Can you work these out from the model? Positions are in its coordinate system, mm. Give positions to 0.01 mm unless a question says otherwise; leave off trailing zeros. Order: outer loops, then holes, each group sorted by start corner. A loop starts at its lowest first (then second) coordinate and runs counter-clockwise, first axis right, second up. Notation, with made-up numbers: (5.5, 26.25) - (61.5, 26.25) arc R21 cw to (61.5, 35.25) - close; hole circle Ø4 at (-39.75, 7). An arc over 180 degrees is marked (long way). Answer as a JSON object with one key per item and string values.
```python
from build123d import *

# Parameters (mm, degrees)
F1_DEPTH = 31.75
F3_D     = 12.7


with BuildPart() as f1:
    # F0 (on Top) → F1 (new body)
    with BuildSketch(Plane.XY):
        with BuildLine():
            Line((45.9964759648, 36.0500998795), (-9.8253758624, 36.0500998795))
            add(Edge.make_bspline(
                [(-42.9035240352, 4.3000998795), (-34.7231067307, 4.914947889), (-18.4671684559, 14.0682512449), (-11.2220877593, 28.5159185869), (-9.8253758624, 36.0500998795)],
                knots=[0, 0, 0, 0, 0.5112036525, 1, 1, 1, 1], degree=3))
            Line((-42.9035240352, 4.3000998795), (-42.9035240352, -27.4499001205))
            Line((-42.9035240352, -27.4499001205), (-22.798109327, -27.4499001205))
            Line((-22.798109327, -27.4499001205), (45.9964759648, 20.0334768742))
            Line((45.9964759648, 20.0334768742), (45.9964759648, 36.0500998795))
        make_face()
    extrude(amount=F1_DEPTH)

    # F3 (through all)
    with Locations(Plane(origin=(-42.9035240352, 0, 0), x_dir=(0, -1, 0), z_dir=(-1, 0, 0))):
        with Locations((11.5749001205, 15.875)):
            Hole(F3_D / 2)


solid = f1.part
```
Q1. If we section it at A-A, the plane x = 31: Please give me the cut outline in (y, z).
Recorded:
{"outline": "(9.68, 0) - (36.05, 0) - (36.05, 31.75) - (9.68, 31.75) - close"}
Q2. I need wall thicknesses on L1, parallel to Z at x = -23, y = -8.5; L2, parallel to Z at x = -29, y = -11; L3, parallel to Y at x = -9, z = 6. Which ranges of each line are inside material? Lowest first, please.
Recorded:
{"L1": "z = 0 to 10.32, 21.43 to 31.75", "L2": "z = 0 to 9.55, 22.2 to 31.75", "L3": "y = -17.93 to 36.05"}
Q3. We'd pull the mould along Z, two halves only. Please class faces 1 (the face through (18, 36.05, 16)), 2 (the face through (-22.196, -5.518, 17.782)), 3 (the face through (1, 5, 0)), 4 (the face through (1, 5, 31.75)): released by +Z, released by -Z, zero draft, split by the parting line, or undercut.
Recorded:
{"face 1": "zero draft", "face 2": "undercut", "face 3": "released by -Z", "face 4": "released by +Z"}
Q4. I'm going to push flat-ended pins straight in: pin 1 Ø3 at (y, z) = (5.5, 12.5) entering from +X; pin 2 Ø2 at (x, z) = (-14, 3.5) entering from -Y; pin 3 Ø16.5 at (y, z) = (-11.57, 15.88) entering from +X; pin 4 Ø10 at (y, z) = (-16.5, 12.5) entering from -X. Where does each tip first touch, or does it pass through?
Recorded:
{"pin 1": "stops at x = 27.11", "pin 2": "stops at y = -22.07", "pin 3": "stops at x = 12.16", "pin 4": "stops at x = -42.9"}
Q5. If we section it at B-B, the plane y = 2.5: Please give me the cut outline in (x, z).
Recorded:
{"outline": "(-42.9, 0) - (20.59, 0) - (20.59, 31.75) - (-42.9, 31.75) - close"}
